from build123d import *

# Parameters (mm, degrees)
SKETCH2_W          = 5
SKETCH2_H          = 1
CUT_EXTRUDE1_DEPTH = 15
SKETCH3_W          = 0.7
SKETCH3_H          = 0.8


with BuildPart() as part:
    # Sketch1 → Revolve1 (revolve)
    with BuildSketch(Plane.XY, mode=Mode.PRIVATE) as revolve1_sk:
        with BuildLine():
            Line((0, 0.5), (7.5, 0.5))
            Line((7.5, 0.5), (7.5, 2))
            Line((7.5, 2), (17.5, 2))
            Line((17.5, 2), (18.928148007, 3))
            ThreePointArc((18.928148007, 3), (27.342618843, 3.065113029), (35.5, 1))
            Line((35.5, 1), (37, 1))
            Line((37, 1), (37, 0))
            Line((37, 0), (36.5, 0))
            Line((36.5, 0), (36.5, 0.5))
            Line((36.5, 0.5), (35.404554146, 0.5))
            ThreePointArc((35.404554146, 0.5), (27.389609996, 2.555633943), (19.115328234, 2.520677712))
            Line((19.115328234, 2.520677712), (17.657649394, 1.5))
            Line((17.657649394, 1.5), (8, 1.5))
            Line((8, 1.5), (8, 0))
            Line((8, 0), (0, 0))
            Line((0, 0), (0, 0.5))
        make_face()
    revolve(revolve1_sk.sketch.rotate(Axis((0, 0, 0), (0, 1, 0)), 90), axis=Axis((0, 0, 0), (0, 1, 0)))

    # Sketch2 → Cut-Extrude1 (cut, symmetric)
    with BuildSketch(Plane.XY):
        with Locations((0, 1)):
            Rectangle(SKETCH2_W, SKETCH2_H)
    extrude(amount=CUT_EXTRUDE1_DEPTH, both=True, mode=Mode.SUBTRACT)

    # Sketch3 → Revolve2 (revolve)
    with BuildSketch(Plane.XY, mode=Mode.PRIVATE) as revolve2_sk:
        with Locations((0.35, 0.9)):
            Rectangle(SKETCH3_W, SKETCH3_H)
    revolve(revolve2_sk.sketch.rotate(Axis((0, 0.5, 0), (0, 1, 0)), 90), axis=Axis((0, 0.5, 0), (0, 1, 0)))


solid = part.part
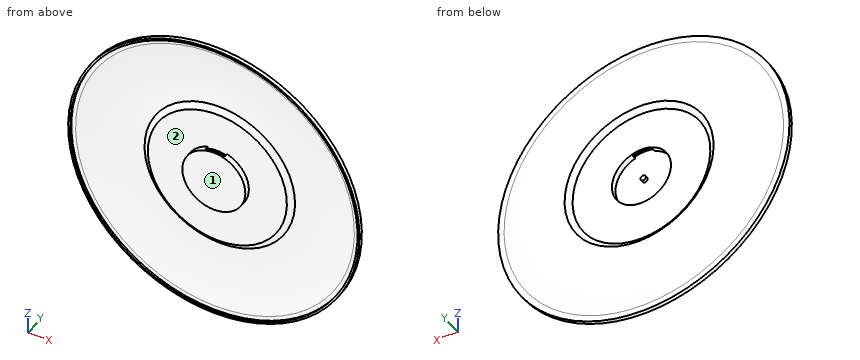
Can you work these out from the model? Positions are in its coordinate system, mm. Face numbers are marked on the shaded views. Round coordinates to 2 decimals unless told otherwise and drop trailing zeros. Use a Markdown table: item, result.
Item 1: If I drill on line 1 along X through (y, z) = (0.2, 0); line 2 along Y through (x, z) = (13, 8); line 3 along Y through (x, z) = (17.5, 15), over which ranges is the centre line in solid material (lowest first)? Write a range as [from, to].
Found:
| item | result |
|---|---|
| line 1 | x = [-37, -36.5], [-8, 8], [36.5, 37] |
| line 2 | y = [1.5, 2] |
| line 3 | y = [2.8, 3.3] |
Item 2: We'd pull the mould along Z, two halves only. Please class the marked faces 1 and 2: released by +Z, released by -Z, zero draft, split by the parting line, or undercut.
Found:
| item | result |
|---|---|
| face 1 | zero draft |
| face 2 | undercut |
Item 3: For pin 1 Ø24 at (x, z) = (0, 0) entering from +Y; pin 2 Ø4 at (x, z) = (26, 15) entering from -Y; pin 3 Ø2 at (x, z) = (22.5, -3) entering from +Y, each with a flat end and sliding along its axis, tell me the tip position at first contact or that it passes through.
Found:
| item | result |
|---|---|
| pin 1 | stops at y = 2 |
| pin 2 | stops at y = 1.64 |
| pin 3 | stops at y = 3.3 |
